Can you work these out from the model? Positions are in its coordinate system, mm. A direction names the side the tool comes from. Give positions to 0.01 mm unless a question says otherwise; leave off trailing zeros. Write each loop counter-clockwise with the first axis right and the second up, starting at its lowest first coordinate (ties: lowest second). Pieces come first, ordered by that corner, then holes. Notation, with made-up numbers: (77.25, 13.25) -> (94.25, 13.25) arc R19 cw to (94.25, 25.25) -> close; hole circle Ø9 at (17, 87). An arc over 180 degrees is marked (long way). Answer as CSV lines item,"result". Start each with the question number.
1. If we section it at D-D on y = 5.5: Write out the boundary of the cut face in (x, z).
2. On a 3-axis mill with a long thin cutter (end or side, diameter ignored), from which of +Z, -Z, +X, -X, +Y, -Y can I reach the whole of each face in a straight line? I mean faces 1 (the face through (31.54, 45.56, -9.39)), 2 (the face through (-31.54, 40.04, -9.39)), 3 (the face through (-31.54, -45.56, -9.39)). Say none if no direction works.
3. I'm going to push flat-ended pins straight in: P1, Ø1.5, axis at x = 13.5, y = -33.5, coming from the -Z side; P2, Ø5, axis at x = 26.5, z = -14, coming from the -Y side; P3, Ø13, axis at x = 19, y = 41, coming from the +Z side; P4, Ø0.7, axis at x = -32, y = -45.5, coming from the -Z side. Where does each tip first touch, or does it pass through?
4. If we section it at C-C on x = -23.5: Write out the boundary of the cut face in (y, z), plus the area to 3 significant figures.
5. I need wall thicknesses on line 1 (X direction, y = 43.5, z = -1.5); line 2 (Y direction, x = 26, z = 8.5); line 3 (Z direction, x = -25, y = 30). Which ranges of each line are inside material? Lowest first, please. Write a range as [from, to].
6. If we mould it in two halves opening along Y, with no side actions, what happens to faces 4 (the face through (12, 45.974, 6)), 5 (the face through (-28.407, 45.561, -9.392)), 6 (the face through (33.147, 7, 1.7))? For each: pulls with the +Y half, pulls with the -Y half, needs draft (parallel to the pull), parting line crosses it, or undercut.
7. If we section it at B-B on x = 16: Write out the boundary of the cut face in (y, z), plus the area to 3 significant figures.
8. If we section it at A-A on z = 3.5: Write out the boundary of the cut face in (x, y), plus the area to 3 significant figures.
```python
from build123d import *

# Parameters (mm, degrees)
F0_W     = 66.294
F0_H     = 91.948
F1_DEPTH = 2.032
F2_W     = 15.24
F2_H     = 11.938
F3_DEPTH = 15.24
F4_R     = 1.5875
F5_DEPTH = 20.32
F6_R     = 8.89
F7_DEPTH = 15.24
F9_DEPTH = 19.05


with BuildPart() as f1:
    # F0 (on Top) → F1 (new body)
    with BuildSketch(Plane.XY):
        Rectangle(F0_W, F0_H)
    extrude(amount=F1_DEPTH)

    # F2 (on face) → F3 (join)
    with BuildSketch(Plane.XY.offset(2.032)):
        with Locations((19.177, 40.005)):
            Rectangle(F2_W, F2_H)
    extrude(amount=F3_DEPTH)

    # F4 (on face) → F5 (join)
    with BuildSketch(Plane(origin=(0, 45.974, 0), x_dir=(-1, 0, 0), z_dir=(0, 1, 0))):
        with Locations((-19.177, 11.176)):
            Circle(F4_R)
    extrude(amount=F5_DEPTH)

    # F6 (on face) → F7 (join)
    with BuildSketch(Plane(origin=(0, 66.294, 0), x_dir=(-1, 0, 0), z_dir=(0, 1, 0))):
        with Locations((-19.177, 11.176)):
            Circle(F6_R)
    extrude(amount=-F7_DEPTH)

    # F8 (on face) → F9 (join)
    with BuildSketch(Plane(origin=(0, 0, 0), x_dir=(1, 0, 0), z_dir=(0, 0, -1))):
        Polygon((33.147, 40.965913), (33.147, 44.632087), (29.972, 46.465174), (26.797, 44.632087), (26.797, 40.965913), (29.972, 39.132826), align=None)
        Polygon((-29.972, 46.465174), (-33.147, 44.632087), (-33.147, 40.965913), (-29.972, 39.132826), (-26.797, 40.965913), (-26.797, 44.632087), align=None)
        Polygon((26.797, -44.632087), (29.972, -46.465174), (33.147, -44.632087), (33.147, -40.965913), (29.972, -39.132826), (26.797, -40.965913), align=None)
        Polygon((-33.147, -40.965913), (-33.147, -44.632087), (-29.972, -46.465174), (-26.797, -44.632087), (-26.797, -40.965913), (-29.972, -39.132826), align=None)
    extrude(amount=F9_DEPTH)


solid = f1.part
```
Computed values:
1,outline,"(-33.15, 0) -> (33.15, 0) -> (33.15, 2.03) -> (-33.15, 2.03) -> close"
2,face 1,"-Z, +X, +Y"
2,face 2,"-Z, -X"
2,face 3,"-Z, -X, -Y"
3,P1,"stops at z = 0"
3,P2,"stops at y = -45.9"
3,P3,"stops at z = 17.27"
3,P4,"stops at z = -19.05"
4,outline,"(-45.97, 0) -> (45.97, 0) -> (45.97, 2.03) -> (-45.97, 2.03) -> close"
4,area,"187 mm2"
5,line 1,"x = [-33.15, -26.8], [26.8, 33.15]"
5,line 2,"y = [34.04, 45.97], [51.05, 66.29]"
5,line 3,"z = [0, 2.03]"
6,face 4,"undercut"
6,face 5,"pulls with the +Y half"
6,face 6,"needs draft"
7,outline,"(-45.97, 0) -> (45.97, 0) -> (45.97, 17.27) -> (34.04, 17.27) -> (34.04, 2.03) -> (-45.97, 2.03) -> close; (51.05, 2.87) -> (66.29, 2.87) -> (66.29, 19.48) -> (51.05, 19.48) -> close"
7,area,"622 mm2"
8,outline,"(11.56, 34.04) -> (26.8, 34.04) -> (26.8, 45.97) -> (11.56, 45.97) -> close; (14.69, 51.05) -> (23.66, 51.05) -> (23.66, 66.29) -> (14.69, 66.29) -> close"
8,area,"319 mm2"
